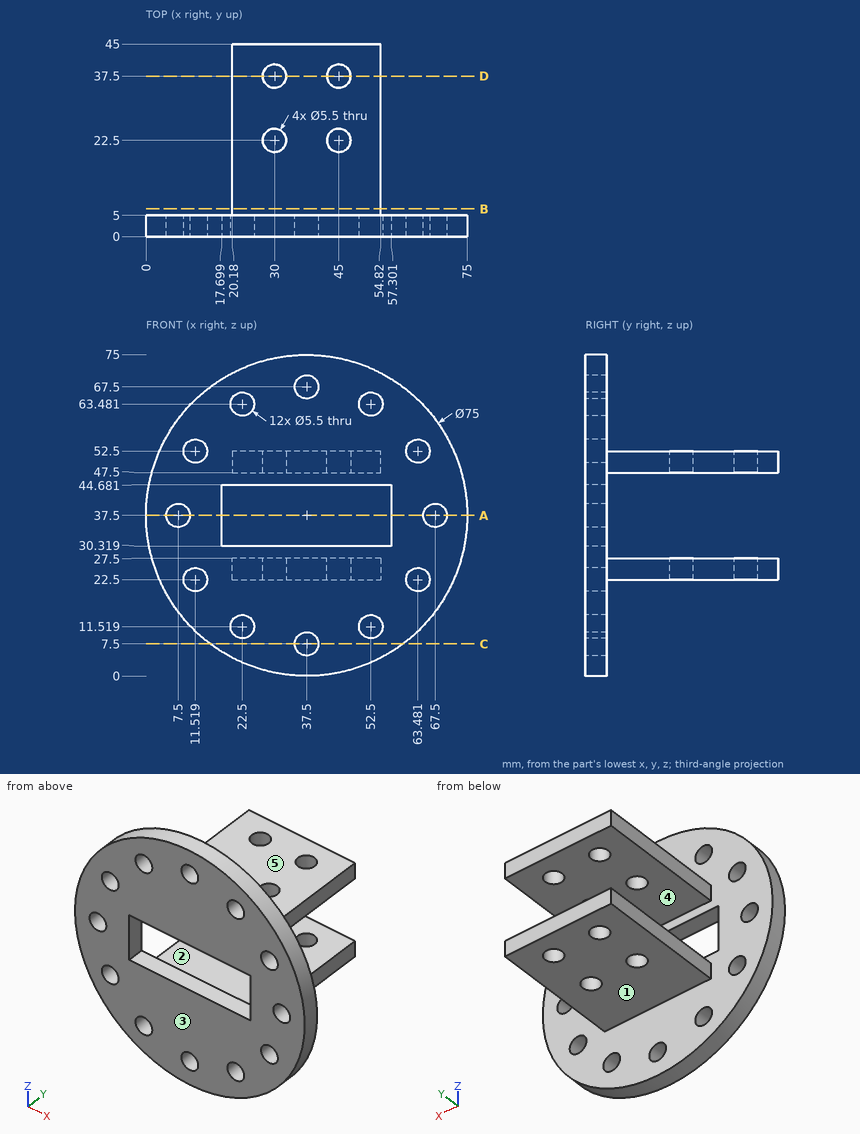
The figure shows three views and two pictorial views of one solid part (mm, origin at its lowest corner). Answer the questions. A direction names the side the tool comes from. Give positions to 0.01 mm unless a question says otherwise; leave off trailing zeros. Order: outer loops, then holes, each group sorted by start corner. A loop starts at its lowest first (then second) coordinate and runs counter-clockwise, first axis right, second up. Notation, with made-up numbers: M -36.75,41.5 L -22.75,41.5 A18 ccw -22.75,64.5 Z; hole C -30,-14 d2. An arc over 180 degrees is marked long. Return JSON: item names as keys, results as strings.
Q1. Which of the six approach directions +Z, -Z, +X, -X, +Y, -Y give full straight-line access (tool end or side, diameter ignored) to the marked faces 4 and 5?
Answer below:
{"face 4": "+X, -X, +Y", "face 5": "+Z, +X, -X, +Y"}
Q2. Each of these flat-tipped pins is pushed along its axis until it touches: pin 1 (7 mm diameter, centred on x = 45, y = 22.5, fed in from -Z); pin 2 (12 mm diameter, centred on x = 38, z = 14.5, fed in from +Y); pin 3 (4.5 mm diameter, centred on x = 45, y = 37.5, fed in from +Z); pin 4 (5.5 mm diameter, centred on x = 31, y = 3, fed in from +Z). Where does it stop, or does it pass through?
Answer below:
{"pin 1": "stops at z = 22.5", "pin 2": "stops at y = 5", "pin 3": "passes through", "pin 4": "stops at z = 74.81"}
Q3. Find section C-C, the plane z = 7.5. Write down the section's boundary in (x, y).
Answer below:
{"outline": "M 15,0 L 34.75,0 L 34.75,5 L 15,5 Z; M 40.25,0 L 60,0 L 60,5 L 40.25,5 Z"}
Q4. Find section B-B, the plane y = 6.5. Write down the section's boundary in (x, z).
Answer below:
{"outline": "M 20.18,22.5 L 54.82,22.5 L 54.82,27.5 L 20.18,27.5 Z; M 20.18,47.5 L 54.82,47.5 L 54.82,52.5 L 20.18,52.5 Z"}
Q5. Find section A-A, the plane z = 37.5. Write down the section's boundary in (x, y), and give its area (3 significant figures).
Answer below:
{"outline": "M 0,0 L 4.75,0 L 4.75,5 L 0,5 Z; M 10.25,0 L 17.7,0 L 17.7,5 L 10.25,5 Z; M 57.3,0 L 64.75,0 L 64.75,5 L 57.3,5 Z; M 70.25,0 L 75,0 L 75,5 L 70.25,5 Z", "area": "122 mm^2"}
Q6. Find the intervals of material crossed by line 1 along X through (y, z) = (22.5, 49.8); line 2 along Z through (x, y) = (40.5, 32.5); line 3 along Y through (x, z) = (30, 25), in increasing order. Write a range as [from, to].
Answer below:
{"line 1": "x = [20.18, 27.25], [32.75, 42.25], [47.75, 54.82]", "line 2": "z = [22.5, 27.5], [47.5, 52.5]", "line 3": "y = [0, 19.75], [25.25, 34.75], [40.25, 45]"}
Q7. Find section D-D, the plane y = 37.5. Write down the section's boundary in (x, z).
Answer below:
{"outline": "M 20.18,22.5 L 27.25,22.5 L 27.25,27.5 L 20.18,27.5 Z; M 20.18,47.5 L 27.25,47.5 L 27.25,52.5 L 20.18,52.5 Z; M 32.75,22.5 L 42.25,22.5 L 42.25,27.5 L 32.75,27.5 Z; M 32.75,47.5 L 42.25,47.5 L 42.25,52.5 L 32.75,52.5 Z; M 47.75,22.5 L 54.82,22.5 L 54.82,27.5 L 47.75,27.5 Z; M 47.75,47.5 L 54.82,47.5 L 54.82,52.5 L 47.75,52.5 Z"}
Q8. The mould has two halves that part along Z. Classify the marked faces 1, 2 and 3: pulls with the +Z half, pulls with the -Z half, needs draft (parallel to the pull), parting line crosses it, or undercut.
Answer below:
{"face 1": "pulls with the -Z half", "face 2": "undercut", "face 3": "needs draft"}
